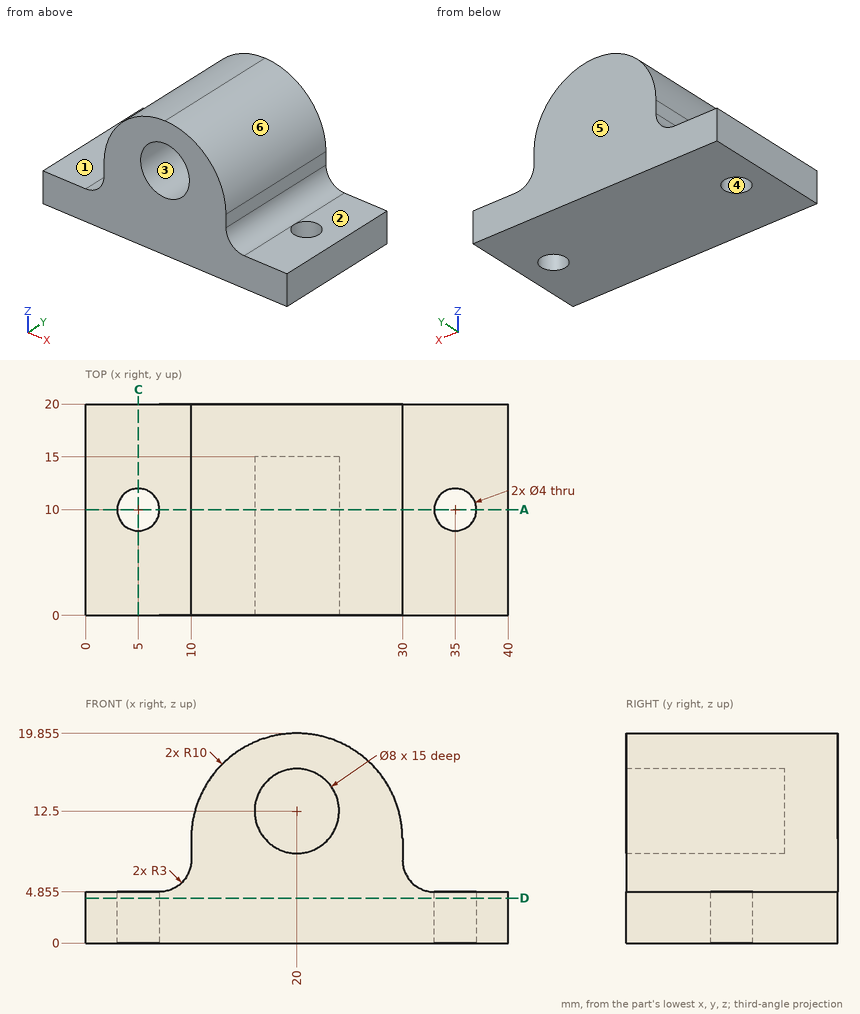
Design review of the part shown in the three views and the two pictorial views. Dimensions are in mm from the part's minimum x, y and z. A direction names the side the tool comes from. Round coordinates to 2 decimals unless told otherwise and drop trailing zeros. Write each loop counter-clockwise with the first axis right and the second up, starting at its lowest first coordinate (ties: lowest second). Pieces come first, ordered by that corner, then holes.
Item 1: We need section C-C on x = 5. Write out the cut boundary in (y, z) (1 decimal), and give its area (3 significant figures).
Item 2: The part is to be moulded in two halves that separate along Y. For the marked faces 4, 5 and 6, say which applies: +Y half, -Y half, draft (parallel to the pull), parting line (faces both ways), or undercut.
Item 3: We need section A-A on y = 10. State how many separate pieces and enclosed holes the cut face has, and give its area (3 significant figures).
Item 4: Clearance check with flat-ended pins moving along their axes: pin 1 Ø1 at (y, z) = (7, 9) entering from -X; pin 2 Ø1.5 at (x, y) = (21, 16) entering from +Z; pin 3 Ø3 at (y, z) = (13.5, 7.5) entering from -X. State where each tip first meets the part, or that it passes through.
Item 5: We need section D-D on z = 4.25. Write out the cut boundary in (x, y).
Item 6: For probe 1 along Y at (x, z) = (35, 1.95); probe 2 along Y at (x, z) = (22, 13.75); probe 3 along Z at (x, y) = (2, 3.25) (1 decimal), list the stretches that pass through material, from the lowest coordinate up.
Item 7: For the marked faces 1, 2 and 3, list the 3-axis set-ups (+Z, -Z, +X, -X, +Y, -Y) from which the entire face can be reached by the end or side of a thin tool; tool diameter is ignored.
Returned:
1. outline: (0, 0) - (8, 0) - (8, 4.9) - (0, 4.9) - close; (12, 0) - (20, 0) - (20, 4.9) - (12, 4.9) - close
1. area: 77.7 mm2
2. face 4: undercut
2. face 5: +Y half
2. face 6: draft
3. separate pieces: 3
3. enclosed holes: 1
3. area: 366 mm2
4. pin 1: stops at x = 10
4. pin 2: stops at z = 19.85
4. pin 3: stops at x = 9.36
5. outline: (0, 0) - (40, 0) - (40, 20) - (0, 20) - close; hole circle Ø4 at (5, 10); hole circle Ø4 at (35, 10)
6. probe 1: y = 0 to 8, 12 to 20
6. probe 2: y = 15 to 20
6. probe 3: z = 0 to 4.9
7. face 1: +Z, -X, +Y, -Y
7. face 2: +Z, +X, +Y, -Y
7. face 3: -Y
